from build123d import *

# Parameters (mm, degrees)
F1_DEPTH    = 5.5
F2_W        = 125
F2_H        = 32
F3_DEPTH    = 2
F4_W        = 3.5
F4_H        = 5.5
F4_W_2      = 4
F5_DEPTH    = 125
F6_R        = 1
F7_C1_SIZE2 = 1
F7_C1_SIZE  = 5.6712818196
F7_C2_SIZE2 = 5.6712818196
F7_C2_SIZE  = 1


with BuildPart() as f1:
    # F0 (on Top) → F1 (new body)
    with BuildSketch(Plane.XY):
        Polygon((57.6, -16.5), (62.5, -16.5), (62.5, 15.5), (57.6, 15.5), (57.6, 5), (41.6, 5), (41.6, 15.5), (32.8, 15.5), (32.8, 5), (16.8, 5), (16.8, 15.5), (8, 15.5), (8, 5), (-8, 5), (-8, 15.5), (-16.8, 15.5), (-16.8, 5), (-32.8, 5), (-32.8, 15.5), (-41.6, 15.5), (-41.6, 5), (-57.6, 5), (-57.6, 15.5), (-62.5, 15.5), (-62.5, -16.5), (-57.6, -16.5), (-57.6, -6), (-41.6, -6), (-41.6, -16.5), (-32.8, -16.5), (-32.8, -6), (-16.8, -6), (-16.8, -16.5), (-8, -16.5), (-8, -6), (8, -6), (8, -16.5), (16.8, -16.5), (16.8, -6), (32.8, -6), (32.8, -16.5), (41.6, -16.5), (41.6, -6), (57.6, -6), align=None)
    extrude(amount=F1_DEPTH)

    # F2 (on face) → F3 (join)
    with BuildSketch(Plane(origin=(0, 0, 0), x_dir=(1, 0, 0), z_dir=(0, 0, -1))):
        with Locations((0, 0.5)):
            Rectangle(F2_W, F2_H)
    extrude(amount=F3_DEPTH)

    # F4 (on face) → F5 (cut, through all)
    with BuildSketch(Plane(origin=(-62.5, 0, 0), x_dir=(0, -1, 0), z_dir=(-1, 0, 0))):
        with Locations((-2.75, 0.75)):
            Rectangle(F4_W, F4_H)
        with Locations((3.5, 0.75)):
            Rectangle(F4_W_2, F4_H)
    extrude(amount=-F5_DEPTH, mode=Mode.SUBTRACT)

    # F6
    f6_edges = [f1.edges().sort_by_distance(p)[0] for p in [
        (0, 4.5, -2),
        (0, 1, -2),
        (0, -5.5, -2),
        (0, -1.5, -2),
    ]]
    fillet(f6_edges, radius=F6_R)

    # F7: chamfer of 1 x 5.6712818196 on 12 edges, made by hand

    # F7_c1
    f7_c1_edges = [f1.edges().sort_by_distance(p)[0] for p in [
        (-12.4, -16.5, 5.5),
    ]]
    f7_c1_side = f1.faces().sort_by_distance((-12.4, -16.5, 5.48))[0]
    chamfer(f7_c1_edges, length=F7_C1_SIZE, length2=F7_C1_SIZE2, reference=f7_c1_side)

    # F7_c2
    f7_c2_edges = [f1.edges().sort_by_distance(p)[0] for p in [
        (12.4, 15.5, 5.5),
    ]]
    f7_c2_side = f1.faces().sort_by_distance((12.4, 15.48, 5.5))[0]
    chamfer(f7_c2_edges, length=F7_C2_SIZE, length2=F7_C2_SIZE2, reference=f7_c2_side)


solid = f1.part
For this review, take the finished solid that the model builds, in its own axes (mm). A direction names the side the tool comes from. Give positions to 0.01 mm unless a question says otherwise; leave off trailing zeros. Loops run counter-clockwise (first coordinate to the right, second up) from the corner with the lowest first, then second, coordinate; pieces in that order, holes last.
Item 1: For line 1 along X through (y, z) = (6, 0.5); line 2 along Y through (x, z) = (-26, -0.25); line 3 along Y through (x, z) = (-56.5, 2), list the stretches that pass through material, from the lowest coordinate up.
Item 2: Take a section at C-C, the plane x = -10. State the section outline as (y, z) points.
Item 3: Take a section at B-B, the plane x = 24. State the section outline as (y, z) points.
Item 4: Tool access review of faces 3 (the flat face through (-32.8, 10, 3)), 4 (the flat face through (-1, 10, -2)), 5 (the flat face through (-57.6, -11, 3)), 6 (the flat face through (-1, -3, 3.5)): name each direction out of +Z, -Z, +X, -X, +Y, -Y from which nothing blocks a thin tool from reaching the whole face with its end or side.
Item 5: Draft analysis for pull direction X (two halves, no side actions). For faces 1 (the flat face through (-1, -12, -2)), 2 (the flat face through (-8, -11, 3)), state which applies: +X half, -X half, draft (parallel to the pull), parting line (faces both ways), or undercut.
Item 6: Take a section at D-D, the plane z = 1.5. Give the number of separate pieces and of enclosed holes in the cut face, and give its area (3 significant figures).
Item 7: Insertion check: pin 1 (8.5 mm diameter, centred on x = -51, y = 12, fed in from +Z); pin 2 (4.5 mm diameter, centred on x = -26.5, z = 3, fed in from -Y); pin 3 (1 mm diameter, centred on x = -20.5, y = -2.5, fed in from -Z). Each pin has a flat end and moves straight along its axis. Give the tip position at first contact, or say it passes through.
Item 8: Take a section at A-A, the plane y = 12. State the section outline as (x, z) points.
Calculated:
1. line 1: x = -62.5 to -57.6, -41.6 to -32.8, -16.8 to -8, 8 to 16.8, 32.8 to 41.6, 57.6 to 62.5
1. line 2: y = -16.5 to -5.5, -1.5 to 1, 4.5 to 15.5
1. line 3: y = -6 to -5.5, -1.5 to 1, 4.5 to 5
2. outline: (-16.5, -2) - (-6.5, -2) arc R1 ccw to (-5.5, -1) - (-5.5, 3.5) - (-1.5, 3.5) - (-1.5, -1) arc R1 ccw to (-0.5, -2) - (0, -2) arc R1 ccw to (1, -1) - (1, 3.5) - (4.5, 3.5) - (4.5, -1) arc R1 ccw to (5.5, -2) - (15.5, -2) - (15.5, -0.17) - (14.5, 5.5) - (-15.5, 5.5) - (-16.5, -0.17) - close
3. outline: (-16.5, -2) - (-6.5, -2) arc R1 ccw to (-5.5, -1) - (-5.5, 3.5) - (-1.5, 3.5) - (-1.5, -1) arc R1 ccw to (-0.5, -2) - (0, -2) arc R1 ccw to (1, -1) - (1, 3.5) - (4.5, 3.5) - (4.5, -1) arc R1 ccw to (5.5, -2) - (15.5, -2) - (15.5, -0.17) - (15.47, 0) - (5, 0) - (5, 5.5) - (-6, 5.5) - (-6, 0) - (-16.47, 0) - (-16.5, -0.17) - close
4. face 3: +Z, +Y
4. face 4: -Z, +X, -X, +Y, -Y
4. face 5: +Z, -Y
4. face 6: -Z, +X, -X
5. face 1: draft
5. face 2: undercut
6. separate pieces: 3
6. enclosed holes: 0
6. area: 1,360 mm2
7. pin 1: stops at z = 0
7. pin 2: stops at y = -6
7. pin 3: stops at z = 3.5
8. outline: (-62.5, -2) - (62.5, -2) - (62.5, 5.5) - (57.6, 5.5) - (57.6, 0) - (41.6, 0) - (41.6, 5.5) - (32.8, 5.5) - (32.8, 0) - (16.8, 0) - (16.8, 5.5) - (8, 5.5) - (8, 0) - (-8, 0) - (-8, 5.5) - (-16.8, 5.5) - (-16.8, 0) - (-32.8, 0) - (-32.8, 5.5) - (-41.6, 5.5) - (-41.6, 0) - (-57.6, 0) - (-57.6, 5.5) - (-62.5, 5.5) - close
